Autodesk Inventor part; units mm, degrees
ref_plane "YZ Plane" through (0, 0, 0) normal (1, 0, 0) x (0, 1, 0)
ref_plane "XZ Plane" through (0, 0, 0) normal (0, 1, 0) x (-1, 0, 0)
ref_plane "XY Plane" through (0, 0, 0) normal (0, 0, 1) x (1, 0, 0)
sketch "Sketch1" plane through (0, 0, 0) normal (0, 0, 1) x (1, 0, 0)
  line L0 (-500, 500) -> (500, 500)
  line L1 (500, 500) -> (500, -500)
  line L2 (500, -500) -> (-500, -500)
  line L3 (-500, -500) -> (-500, 500)
  line L4 (-500, 500) -> (500, -500) construction
  line L5 (500, 500) -> (-500, -500) construction
  point P0 (0, 0)
  dimension "d0" = 1000
  dimension "d1" = 1000
extrude "Extrusion1" add sketch "Sketch1" along normal blind 1200 draft -5
fillet "Fillet1" radius 250 8 edges at (447.5068, 447.5068, 600) (-447.5068, 447.5068, 600) (447.5068, -447.5068, 600) (-447.5068, -447.5068, 600) (500, 0, 0) (0, 500, 0) (-500, 0, 0) (0, -500, 0)
properties part number "NDM-VOS dummy Crane"
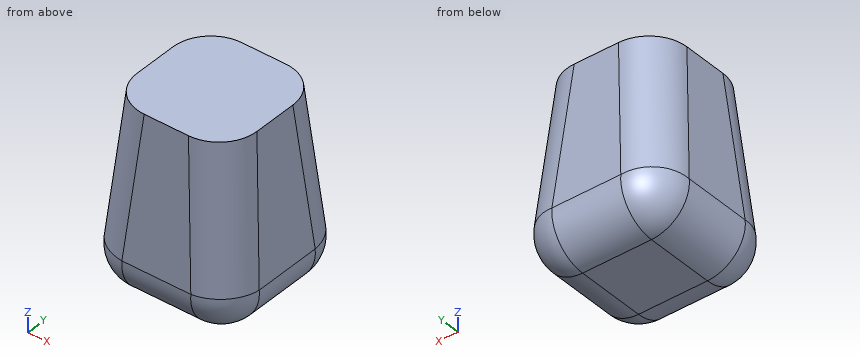
CAD build for the part. Positions are in the model's coordinates, mm. Coordinates: 2 decimals unless noted, no trailing zeros. Write each loop counter-clockwise with the first axis right and the second up, starting at its lowest first coordinate (ties: lowest second). Pieces come first, ordered by that corner, then holes.
(1) Drill centre lines: probe 1 along Z at (x, y) = (-238, -215.5); probe 2 along X at (y, z) = (174, 918); probe 3 along Y at (x, z) = (252, 1136.5). Where is each one in solid material? Low to high.
(2) Flat gauge pins, fed straight in: pin 1 (1.5 mm diameter, centred on x = 249, z = 469.5, fed in from -Y); pin 2 (5 mm diameter, centred on y = 145, z = 520, fed in from +X); pin 3 (10 mm diameter, centred on x = -146.5, z = 674.5, fed in from -Y). Where does each tip first touch, or does it go through?
(3) Cut at B-B, the plane z = 177.5. List the corners of the cut face in (x, y), and give its area (3 significant figures).
(4) Cut at A-A, the plane x = 52.5. List the corners of the cut face in (y, z).
Geometry says:
1. probe 1: z = 0.23 to 1200
1. probe 2: x = -419.66 to 419.66
1. probe 3: y = -379.5 to 379.5
2. pin 1: stops at y = -455.99
2. pin 2: stops at x = 454.72
2. pin 3: stops at y = -441.43
3. outline: (-466.43, -227.17) arc R239.26 ccw to (-227.17, -466.43) - (227.17, -466.43) arc R239.26 ccw to (466.43, -227.17) - (466.43, 227.17) arc R239.26 ccw to (227.17, 466.43) - (-227.17, 466.43) arc R239.26 ccw to (-466.43, 227.17) - close
3. area: 821,000 mm2
4. outline: (-476.22, 271.79) arc R250 ccw to (-227.17, 0) - (227.17, 0) arc R250 ccw to (476.22, 271.79) - (395.01, 1200) - (-395.01, 1200) - close
